Verification items for the finished model (mm, model axes). Face numbers are marked on the shaded views. A direction names the side the tool comes from. Round coordinates to 2 decimals unless told otherwise and drop trailing zeros. Write each loop counter-clockwise with the first axis right and the second up, starting at its lowest first coordinate (ties: lowest second). Pieces come first, ordered by that corner, then holes. Notation, with made-up numbers: M -0.5,29 L 28.5,29 A23 cw 28.5,53 Z; hole C 18.5,-32.5 d8. An arc over 180 degrees is marked long. One line per question, with ' | ' between items.
Autodesk Fusion 360 part; units mm, degrees
sketch "Sketch1" plane through (0, 0, 0) normal (0, 0, 1) x (1, 0, 0)
  line L0 (0, 0) -> (-70, 0)
  line L1 (-70, 0) -> (-70, -37)
  line L2 (-70, -37) -> (0, -37)
  line L3 (0, -37) -> (0, 0)
  line L4 (2, 2) -> (-72, 2)
  line L5 (-72, 2) -> (-72, -39)
  line L6 (-72, -39) -> (2, -39)
  line L7 (2, -39) -> (2, 2)
  dimension "d1" = 37
  dimension "d2" = 70
  dimension "d3" = 2
extrude "Extrude1" add sketch "Sketch1" along normal blind 42
extrude "Extrude2" add sketch "Sketch1" along normal blind 2 contours L0 L1 L2 L3
fillet "Fillet1" radius 1 4 edges at (0, -37, 22) (-70, -37, 22) (-70, 0, 22) (0, 0, 22)
fillet "Fillet2" radius 1 4 edges at (2, -39, 21) (-72, -39, 21) (-72, 2, 21) (2, 2, 21)
chamfer "Chamfer1" distance 1 angle 45 8 edges at (-70, -18.5, 2) (-69.7071, -0.2929, 2) (-35, 0, 2) (-0.2929, -0.2929, 2) (0, -18.5, 2) (-0.2929, -36.7071, 2) (-35, -37, 2) (-69.7071, -36.7071, 2)
sketch "Sketch2" plane through (0, 2, 0) normal (0, 1, 0) x (-1, 0, 0)
  line L0 (-1, 42) -> (-1, 0)
  line L1 (-1, 0) -> (71, 0)
  line L2 (71, 0) -> (71, 42)
  line L3 (71, 42) -> (-1, 42)
  line L4 (35, 42) -> (35, 0) construction
  line L5 (22.2945, 42) -> (22.2945, 15.7055)
  line L6 (47.7055, 42) -> (47.7055, 15.7055)
  arc A0 (22.2945, 15.7055) -> (47.7055, 15.7055) centre (35, 15.7055) ccw
  circle A1 centre (10.6473, 32) radius 4.5
  circle A2 centre (59.3527, 32) radius 4.5
  line L7 (-1, 32) -> (22.2945, 32) construction
  dimension "d13" = 3
  dimension "d14" = 9
  dimension "d15" = 10
extrude "Extrude3" cut sketch "Sketch2" against normal up to surface (2 mm away) contours L3 L5 L6 A0 | A1 | A2
fillet "Fillet3" radius 4 2 edges at (-22.2945, 1, 42) (-47.7055, 1, 42)
sketch "projecting holes for attachment" plane through (0, -37, 0) normal (0, 1, 0) x (-1, 0, 0)
  line L0 (1, 3) -> (69, 3)
  line L1 (69, 3) -> (69, 42)
  line L2 (69, 42) -> (1, 42)
  line L3 (1, 42) -> (1, 3)
  point P0 (10.6473, 32)
  point P1 (59.3527, 32)
hole "Hole1" at (-59.3527, -37, 32) at (-10.6473, -37, 32) direction (0, -1, 0) diameter 5 depth 11 tip angle 118 countersink diameter 8.5 countersink angle 90
sketch "Splitting the base for printability" plane through (2, 0, 0) normal (1, 0, 0) x (0, 1, 0)
  line L0 (1, 0) -> (1, 42)
  line L1 (1, 42) -> (-38, 42)
  line L2 (-38, 42) -> (-38, 0)
  line L3 (-38, 0) -> (1, 0)
  line L4 (-38, 0) -> (1, 0)
  line L5 (-18.5, 0) -> (-18.5, 1) construction
  line L6 (-18.5, 1) -> (-19.5, 0)
  line L7 (-18.5, 1) -> (-17.5, 0)
  dimension "d26" = 1
  dimension "d27" = 90
extrude "Extrude4" cut sketch "Splitting the base for printability" against normal up to surface (74 mm away) contours L3 L4 L6 L7
sketch "Splitting the base for printability 2" plane through (0, -39, 0) normal (0, -1, 0) x (1, 0, 0)
  circle A0 centre (-59.3527, 32) radius 2.5
  circle A1 centre (-10.6473, 32) radius 2.5
  line L0 (-71, 42) -> (-71, 0)
  line L1 (-71, 0) -> (1, 0)
  line L2 (1, 0) -> (1, 42)
  line L3 (1, 42) -> (-71, 42)
  line L4 (-35, 0) -> (-35, 1) construction
  line L5 (-35, 1) -> (-34, 0)
  line L6 (-35, 1) -> (-36, 0)
  dimension "d30" = 1
  dimension "d31" = 90
extrude "Extrude5" cut sketch "Splitting the base for printability 2" against normal blind 41 contours L1 L5 L6
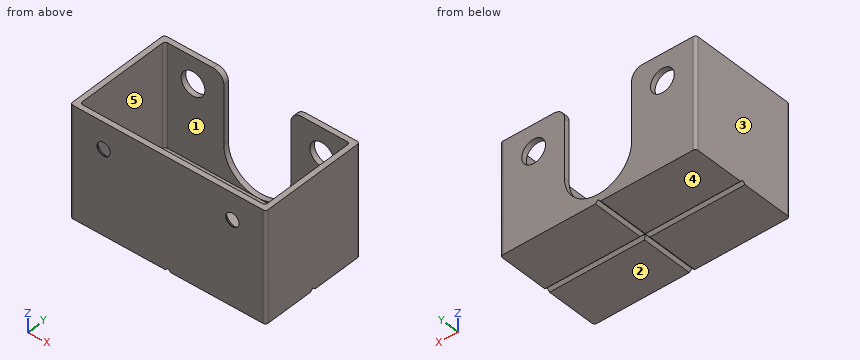
1. Mould release check, pull along X, two halves, no side actions. Record for the marked faces 1, 2 and 3: pulls with the +X half, pulls with the -X half, needs draft (parallel to the pull), parting line crosses it, or undercut.
Results:
face 1: undercut | face 2: needs draft | face 3: pulls with the -X half
2. Thickness scan on line 1 (X direction, y = -23, z = 37); line 2 (Y direction, x = -13, z = 12.5); line 3 (X direction, y = -38.85, z = 32). Record the ranges inside material, lowest first.
Results:
line 1: x = -72 to -70, 0 to 2 | line 2: y = -39 to -37, 0 to 2 | line 3: x = -71.53 to -61.85, -56.85 to -13.15, -8.15 to 1.53
3. Tool access check on the marked faces 4 and 5. Record the directions out of +Z, -Z, +X, -X, +Y, -Y that give a thin tool (end or side, any length) a straight path to the whole face; none if there is none.
Results:
face 4: -Z, +X, -X, +Y, -Y | face 5: +Z
4. Section check D-D, the plane x = -26. Record the cut outline in (y, z), then the cut area to 3 significant figures.
Results:
outline: M -39,0 L -19.5,0 L -18.5,1 L -17.5,0 L 2,0 L 2,6.74 L 0,6.74 L 0,3 L -1,2 L -36,2 L -37,3 L -37,42 L -39,42 Z | area: 171 mm2
5. Section check B-B, the plane z = 32. Count the separate pieces of the cut face and the enclosed holes in it, then the cut area to 3 significant figures.
Results:
separate pieces: 5 | enclosed holes: 0 | area: 331 mm2
6. Section check C-C, the plane y = -25. Record the cut outline in (x, z), then the cut area to 3 significant figures.
Results:
outline: M -72,0 L -36,0 L -35,1 L -34,0 L 2,0 L 2,42 L 0,42 L 0,3 L -1,2 L -69,2 L -70,3 L -70,42 L -72,42 Z | area: 308 mm2
7. Go/stop test with flat-tipped pins: P1, Ø11.5, axis at x = -31.5, z = 19, coming from the +Y side; P2, Ø8, axis at x = -10.65, z = 32, coming from the +Y side; P3, Ø4.5, axis at x = -59.35, z = 32, coming from the -Y side; P4, Ø17.5, axis at x = -38, y = -16.5, coming from the +Z side. Record where each tip stops, or that it passes through.
Results:
P1: stops at y = -37 | P2: stops at y = -37.25 | P3: passes through | P4: stops at z = 2
8. Section check A-A, the plane z = 18. Record the cut outline in (x, y), then the cut area to 3 significant figures.
Results:
outline: M -72,-38 A1 ccw -71,-39 L 1,-39 A1 ccw 2,-38 L 2,1 A1 ccw 1,2 L -22.29,2 L -22.29,0 L -1,0 A1 cw 0,-1 L 0,-36 A1 cw -1,-37 L -69,-37 A1 cw -70,-36 L -70,-1 A1 cw -69,0 L -47.71,0 L -47.71,2 L -71,2 A1 ccw -72,1 Z | area: 393 mm2
